Verification items for the finished model (mm, model axes). A direction names the side the tool comes from. Coordinates: 2 decimals unless noted, no trailing zeros. Write each loop counter-clockwise with the first axis right and the second up, starting at its lowest first coordinate (ties: lowest second). Pieces come first, ordered by that corner, then holes. Notation, with made-up numbers: (74.5, 45.25) -> (89.5, 45.25) arc R27 cw to (89.5, 66.25) -> close; hole circle Ø5 at (30, 15). An arc over 180 degrees is marked (long way). Answer in a Markdown table with one row per item.
```python
from build123d import *

# Parameters (mm, degrees)
SKETCH1_R                       = 72
BOSS_EXTRUDE1_DEPTH             = 2.5
SKETCH2_R                       = 0.75
CUT_EXTRUDE1_DEPTH              = 2.5
SKETCH5_W                       = 40
SKETCH5_H                       = 18
BOSS_EXTRUDE3_DEPTH             = 40
SKETCH6_W                       = 33.5
SKETCH6_H                       = 16.220064856
CUT_EXTRUDE2_DEPTH              = 3.5
SKETCH7_W                       = 23
SKETCH7_H                       = 16.220064856
CUT_EXTRUDE3_DEPTH              = 2
SKETCH8_W                       = 16.5
SKETCH8_H                       = 16.220064856
CUT_EXTRUDE4_DEPTH              = 7
SKETCH9_W                       = 5
SKETCH9_H                       = 40
CUT_EXTRUDE5_DEPTH              = 93
SKETCH10_W                      = 16.5
SKETCH10_H                      = 16.220064856
CUT_EXTRUDE6_DEPTH              = 83.5
SKETCH13_W                      = 33.5
SKETCH13_H                      = 1.36
BOSS_EXTRUDE4_DEPTH             = 9.5
M2X0_4_TAPPED_HOLE1_D           = 1.6
M2X0_4_TAPPED_HOLE1_DEPTH       = 6
M2X0_4_TAPPED_HOLE1_CSINK_D     = 2.05
M2X0_4_TAPPED_HOLE1_CSINK_ANGLE = 90
M2X0_4_TAPPED_HOLE1_TIP         = 0.480688495
FILLET1_R                       = 3
FILLET2_R                       = 3
FILLET3_R                       = 3
SKETCH16_R                      = 6.5
CUT_EXTRUDE7_DEPTH              = 3.5
FILLET4_R                       = 1
SKETCH17_R                      = 0.75
CUT_EXTRUDE8_DEPTH              = 3.5


with BuildPart() as part:
    # Sketch1 → Boss-Extrude1 (new body)
    with BuildSketch(Plane(origin=(0, 0, 0), x_dir=(1, 0, 0), z_dir=(0, 1, 0))):
        Circle(SKETCH1_R)
    extrude(amount=BOSS_EXTRUDE1_DEPTH)

    # Sketch2 → Cut-Extrude1 (cut)
    with BuildSketch(Plane(origin=(0, 0, 0), x_dir=(-1, 0, 0), z_dir=(0, -1, 0))):
        with Locations((-11.25, 0)):
            Circle(SKETCH2_R)
        with Locations((11.25, 0)):
            Circle(SKETCH2_R)
    extrude(amount=-CUT_EXTRUDE1_DEPTH, mode=Mode.SUBTRACT)

    # Sketch5 → Boss-Extrude3 (add)
    with BuildSketch(Plane(origin=(0, 2.5, 0), x_dir=(1, 0, 0), z_dir=(0, 1, 0))):
        with Locations((0, -14)):
            Rectangle(SKETCH5_W, SKETCH5_H)
    extrude(amount=BOSS_EXTRUDE3_DEPTH)

    # Sketch6 → Cut-Extrude2 (cut)
    with BuildSketch(Plane.XY.offset(23)):
        with Locations((0, 29.389629851)):
            Rectangle(SKETCH6_W, SKETCH6_H)
    extrude(amount=-CUT_EXTRUDE2_DEPTH, mode=Mode.SUBTRACT)

    # Sketch7 → Cut-Extrude3 (cut)
    with BuildSketch(Plane.XY.offset(19.5)):
        with Locations((0, 29.389629851)):
            Rectangle(SKETCH7_W, SKETCH7_H)
    extrude(amount=-CUT_EXTRUDE3_DEPTH, mode=Mode.SUBTRACT)

    # Sketch8 → Cut-Extrude4 (cut)
    with BuildSketch(Plane.XY.offset(17.5)):
        with Locations((-3.25, 29.389629851)):
            Rectangle(SKETCH8_W, SKETCH8_H)
    extrude(amount=-CUT_EXTRUDE4_DEPTH, mode=Mode.SUBTRACT)

    # Sketch9 → Cut-Extrude5 (cut, through all)
    with BuildSketch(Plane(origin=(20, 0, 0), x_dir=(0, 0, -1), z_dir=(1, 0, 0))):
        with Locations((-7.5, 22.5)):
            Rectangle(SKETCH9_W, SKETCH9_H)
    extrude(amount=-CUT_EXTRUDE5_DEPTH, mode=Mode.SUBTRACT)

    # Sketch10 → Cut-Extrude6 (cut, through all)
    with BuildSketch(Plane.XY.offset(10.5)):
        with Locations((-3.25, 29.389629851)):
            Rectangle(SKETCH10_W, SKETCH10_H)
    extrude(amount=-CUT_EXTRUDE6_DEPTH, mode=Mode.SUBTRACT)

    # Sketch13 → Boss-Extrude4 (add)
    with BuildSketch(Plane.XY.offset(19.5)):
        with Locations((0, 36.819662279)):
            Rectangle(SKETCH13_W, SKETCH13_H)
        with Locations((0, 21.959597423)):
            Rectangle(SKETCH13_W, SKETCH13_H)
    extrude(amount=-BOSS_EXTRUDE4_DEPTH)

    # M2x0.4 Tapped Hole1
    with Locations(Plane.XY.offset(19.5)):
        with Locations((14.5, 29.389662279), (-14.5, 29.389662279)):
            CounterSinkHole(M2X0_4_TAPPED_HOLE1_D / 2, M2X0_4_TAPPED_HOLE1_CSINK_D / 2, depth=M2X0_4_TAPPED_HOLE1_DEPTH, counter_sink_angle=M2X0_4_TAPPED_HOLE1_CSINK_ANGLE)
            with Locations((0, 0, -(M2X0_4_TAPPED_HOLE1_DEPTH + M2X0_4_TAPPED_HOLE1_TIP / 2))):  # 118° drill point
                Cone(0, M2X0_4_TAPPED_HOLE1_D / 2, M2X0_4_TAPPED_HOLE1_TIP, mode=Mode.SUBTRACT)

    # Fillet1
    fillet1_edges = [part.edges().sort_by_distance(p)[0] for p in [
        (-20, 22.5, 23),
        (20, 22.5, 23),
        (-20, 22.5, 10),
        (20, 22.5, 10),
    ]]
    fillet(fillet1_edges, radius=FILLET1_R)

    # Fillet2
    fillet2_edges = [part.edges().sort_by_distance(p)[0] for p in [
        (20, 2.5, 16.5),
        (0, 2.5, 23),
        (-20, 2.5, 16.5),
        (0, 2.5, 10),
        (19.121320344, 2.5, 22.121320344),
        (-19.121320344, 2.5, 22.121320344),
        (-19.121320344, 2.5, 10.878679656),
        (19.121320344, 2.5, 10.878679656),
    ]]
    fillet(fillet2_edges, radius=FILLET2_R)

    # Fillet3
    fillet3_edges = [part.edges().sort_by_distance(p)[0] for p in [
        (20, 42.5, 16.5),
        (0, 42.5, 23),
        (0, 42.5, 10),
        (-20, 42.5, 16.5),
        (19.121320344, 42.5, 10.878679656),
        (-19.121320344, 42.5, 10.878679656),
        (-19.121320344, 42.5, 22.121320344),
        (19.121320344, 42.5, 22.121320344),
    ]]
    fillet(fillet3_edges, radius=FILLET3_R)

    # Sketch16 → Cut-Extrude7 (cut, through all)
    with BuildSketch(Plane(origin=(0, 2.5, 0), x_dir=(1, 0, 0), z_dir=(0, 1, 0))):
        with Locations((0, -46.614420622)):
            Circle(SKETCH16_R)
    extrude(amount=-CUT_EXTRUDE7_DEPTH, mode=Mode.SUBTRACT)

    # Fillet4
    fillet4_edges = [part.edges().sort_by_distance(p)[0] for p in [
        (-6.5, 0, 46.614420622),
        (-6.5, 2.5, 46.614420622),
    ]]
    fillet(fillet4_edges, radius=FILLET4_R)

    # Sketch17 → Cut-Extrude8 (cut, through all)
    with BuildSketch(Plane(origin=(0, 2.5, 0), x_dir=(1, 0, 0), z_dir=(0, 1, 0))):
        with Locations((4.75, 0)):
            Circle(SKETCH17_R)
        with Locations((-4.75, 0)):
            Circle(SKETCH17_R)
    extrude(amount=-CUT_EXTRUDE8_DEPTH, mode=Mode.SUBTRACT)


solid = part.part
```
1. Sectioned sample at C-C, the plane z = -52. Record the cut outline in (x, y), and give its area (3 significant figures).
Findings below:
| item | result |
|---|---|
| outline | (-49.8, 0) -> (49.8, 0) -> (49.8, 2.5) -> (-49.8, 2.5) -> close |
| area | 249 mm² |
2. Sectioned sample at D-D, the plane x = 39.5. Record the cut outline in (y, z).
Findings below:
| item | result |
|---|---|
| outline | (0, -60.2) -> (2.5, -60.2) -> (2.5, 60.2) -> (0, 60.2) -> close |
3. Go/stop test with flat-tipped pins: pin 1 (1 mm diameter, centred on y = 37, z = 11.5, fed in from -X); pin 2 (2 mm diameter, centred on x = -14.5, y = 29.39, fed in from -Z); pin 3 (2 mm diameter, centred on x = 14.5, y = 29.39, fed in from +Z); pin 4 (10.5 mm diameter, centred on x = 2, z = 14.5, fed in from -Y). Record where each tip stops, or that it passes through.
Findings below:
| item | result |
|---|---|
| pin 1 | stops at x = -19.83 |
| pin 2 | stops at z = 10 |
| pin 3 | stops at z = 19.48 |
| pin 4 | stops at y = 0 |
4. Access from +Z, -Z, +X, -X, +Y, -Y to the whole of each face (thin tool, end or side, straight path). Record for faces 5 (the face through (0, 15, 23)), 6 (the face through (20, 22, 17)), 7 (the face through (16.75, 29, 21)), 8 (the face through (-11.5, 29, 15)).
Findings below:
| item | result |
|---|---|
| face 5 | +Z, +X, -X, +Y |
| face 6 | +Z, -Z, +X, +Y |
| face 7 | +Z |
| face 8 | +Z, -Z |
5. Sectioned sample at B-B, the plane y = 16. Record the cut outline in (x, z), and give its area (3 significant figures).
Findings below:
| item | result |
|---|---|
| outline | (-20, 13) arc R3 ccw to (-17, 10) -> (17, 10) arc R3 ccw to (20, 13) -> (20, 20) arc R3 ccw to (17, 23) -> (-17, 23) arc R3 ccw to (-20, 20) -> close |
| area | 512 mm² |
6. Material ranges on probe 1 along Y at (x, z) = (-14.5, 16.05); probe 2 along Z at (x, y) = (4.75, 1); probe 3 along Y at (x, z) = (-4, -62), recorded low to high. Write a range as from..to.
Findings below:
| item | result |
|---|---|
| probe 1 | y = 0..28.59, 30.19..42.5 |
| probe 2 | z = -71.84..-0.75, 0.75..42.18, 51.05..71.84 |
| probe 3 | y = 0..2.5 |
7. Sectioned sample at A-A, the plane x = 0. Record the cut outline in (y, z).
Findings below:
| item | result |
|---|---|
| outline | (0, -72) -> (2.5, -72) -> (2.5, 7) arc R3 cw to (5.5, 10) -> (22.64, 10) -> (22.64, 19.5) -> (21.28, 19.5) -> (21.28, 23) -> (5.5, 23) arc R3 cw to (2.5, 26) -> (2.5, 39.11) arc R1 ccw to (1.5, 40.11) -> (1, 40.11) arc R1 ccw to (0, 39.11) -> close; (0, 54.11) arc R1 ccw to (1, 53.11) -> (1.5, 53.11) arc R1 ccw to (2.5, 54.11) -> (2.5, 72) -> (0, 72) -> close; (36.14, 10) -> (39.5, 10) arc R3 ccw to (42.5, 13) -> (42.5, 20) arc R3 ccw to (39.5, 23) -> (37.5, 23) -> (37.5, 19.5) -> (36.14, 19.5) -> close |
8. Release check for a two-part mould opening along X. For faces 1 (the face through (-16.75, 29, 21)), 2 (the face through (-20, 22, 17)), 3 (the face through (-1, 0, -1)), 4 (the face through (5, 29, 14)) record: released by +X, released by -X, zero draft, split by the parting line, or undercut.
Findings below:
| item | result |
|---|---|
| face 1 | undercut |
| face 2 | released by -X |
| face 3 | zero draft |
| face 4 | undercut |
